For this review, use the dimensioned drawing (mm, ordinates from the lowest corner) and the shaded views. Coordinates: 2 decimals unless noted, no trailing zeros. Write each loop counter-clockwise with the first axis right and the second up, starting at its lowest first coordinate (ties: lowest second). Pieces come first, ordered by that corner, then holes. Notation, with made-up numbers: (55, -8.5) - (82, -8.5) arc R15 cw to (82, 11.5) - close; hole circle Ø1 at (35.5, -40). An arc over 180 degrees is marked (long way). Answer as a JSON object with one key per item and string values.
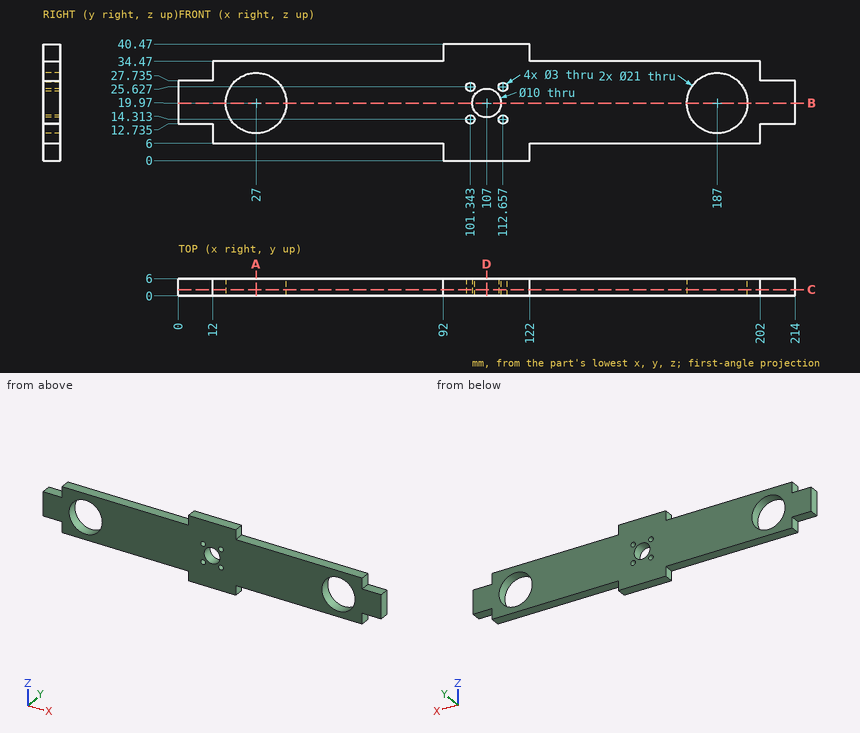
(1) For pin 1 (3 mm diameter, centred on x = 142, y = 4.5, fed in from -Z); pin 2 (1.8 mm diameter, centred on x = 205, y = 4, fed in from +Z) (3 decimals); pin 3 (3 mm diameter, centred on x = 149, y = 1.5, fed in from +Z), all flat-tipped, find the tip position at first contact; note any pin that passes through.
Solved:
{"pin 1": "stops at z = 6", "pin 2": "stops at z = 27.735", "pin 3": "stops at z = 34.47"}
(2) To check wall thickness, follow line 1 (Z direction, x = 107, y = 3.65); line 2 (X direction, y = 0.65, z = 23); line 3 (Z direction, x = 27, y = 1.9). State the ranges of each line that lie inside material, in increasing order. Write a range as from..to.
Solved:
{"line 1": "z = 0..14.97, 24.97..40.47", "line 2": "x = 0..16.95, 37.05..103.02, 110.98..176.95, 197.05..214", "line 3": "z = 6..9.47, 30.47..34.47"}
(3) Take a section at D-D, the plane x = 107. Write out the cut boundary in (y, z), and give its area (3 significant figures).
Solved:
{"outline": "(0, 0) - (6, 0) - (6, 14.97) - (0, 14.97) - close; (0, 24.97) - (6, 24.97) - (6, 40.47) - (0, 40.47) - close", "area": "183 mm^2"}
(4) Take a section at C-C, the plane y = 2.15. Write out the cut boundary in (x, z) (3 decimals), and give its area (3 significant figures).
Solved:
{"outline": "(0, 12.735) - (12, 12.735) - (12, 6) - (92, 6) - (92, 0) - (122, 0) - (122, 6) - (202, 6) - (202, 12.735) - (214, 12.735) - (214, 27.735) - (202, 27.735) - (202, 34.47) - (122, 34.47) - (122, 40.47) - (92, 40.47) - (92, 34.47) - (12, 34.47) - (12, 27.735) - (0, 27.735) - close; hole circle Ø21 at (27, 19.97); hole circle Ø3 at (101.343, 14.313); hole circle Ø3 at (101.343, 25.627); hole circle Ø10 at (107, 19.97); hole circle Ø3 at (112.657, 14.313); hole circle Ø3 at (112.657, 25.627); hole circle Ø21 at (187, 19.97)", "area": "5,330 mm^2"}
(5) Take a section at B-B, the plane z = 19.97. Write out the cut boundary in (x, y), and give its area (3 significant figures).
Solved:
{"outline": "(0, 0) - (16.5, 0) - (16.5, 6) - (0, 6) - close; (37.5, 0) - (102, 0) - (102, 6) - (37.5, 6) - close; (112, 0) - (176.5, 0) - (176.5, 6) - (112, 6) - close; (197.5, 0) - (214, 0) - (214, 6) - (197.5, 6) - close", "area": "972 mm^2"}
(6) Take a section at A-A, the plane x = 27. Write out the cut boundary in (y, z).
Solved:
{"outline": "(0, 6) - (6, 6) - (6, 9.47) - (0, 9.47) - close; (0, 30.47) - (6, 30.47) - (6, 34.47) - (0, 34.47) - close"}
